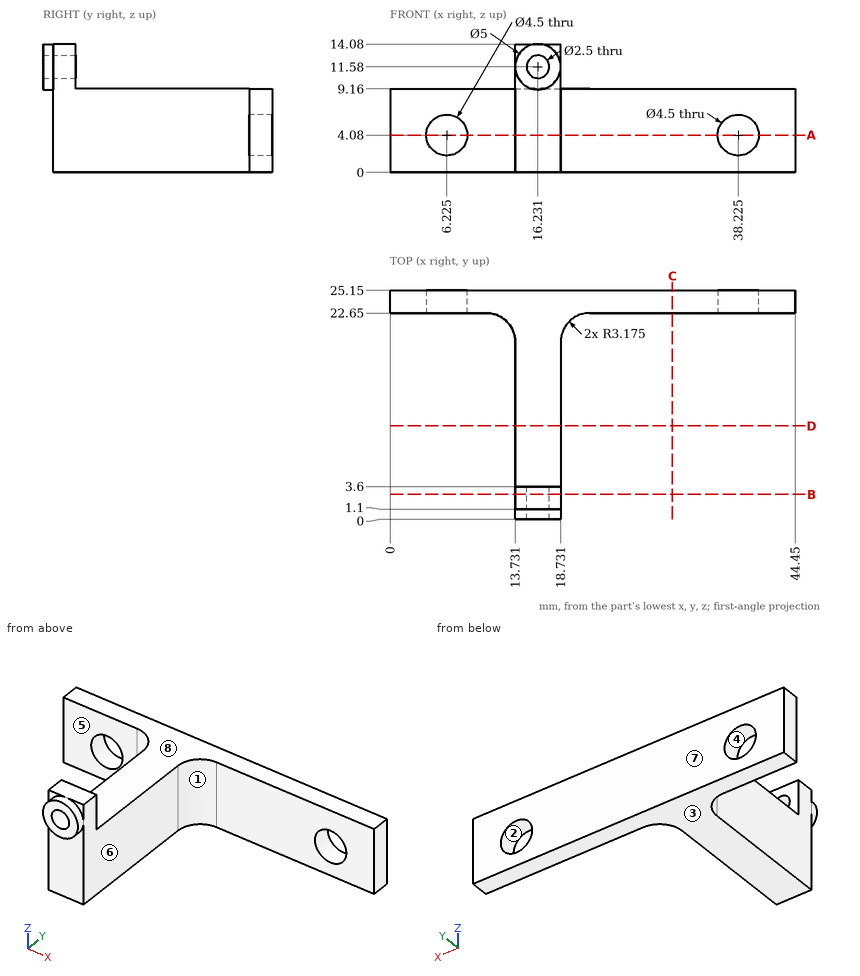
Study the drawing (mm; zero at the part's minimum x, y, z) and answer. A direction names the side the tool comes from. Round coordinates to 2 decimals unless told otherwise and drop trailing zeros. Loops run counter-clockwise (first coordinate to the right, second up) from the corner with the lowest first, then second, coordinate; pieces in that order, holes last.
Q1. Section D-D, the plane y = 10.25 is taken. Determine the outline of the cut face in (x, z).
Q2. Which of the six approach directions +Z, -Z, +X, -X, +Y, -Y give full straight-line access (tool end or side, diameter ignored) to the marked faces 4, 5, 6, 7 and 8?
Q3. Section C-C, the plane x = 31 is taken. Determine the outline of the cut face in (y, z).
Q4. Section A-A, the plane z = 4.08 is taken. Count the separate pieces of the cut face and the enclosed holes in it, then the cut area to 3 significant figures.
Q5. Section B-B, the plane y = 2.75 is taken. Determine the outline of the cut face in (x, z), then the cut area to 3 significant figures.
Q6. Find the intervals of material crossed by line 1 (Y direction, x = 41.5, z = 8.25); line 2 (Z direction, x = 38, y = 23); line 3 (X direction, y = 5, z = 1), in increasing order.
Q7. For a pull along Z with two mould halves and no side action, classify the marked faces 1, 2 and 3 as released by +Z, released by -Z, zero draft, split by the parting line, or undercut.
Q8. Given pin 1 Ø1.5 at (x, z) = (16.23, 11.58) entering from -Y; pin 2 Ø6 at (x, z) = (38.225, 4.08) entering from +Y; pin 3 Ø4 at (x, z) = (16.5, 6.5) entering from -Y; pin 4 Ø7 at (y, z) = (10.5, 4.5) entering from +X, each flat-ended and moving along its own axis, determine where each tip first touches the part or whether it passes through.
Completed:
1. outline: (13.73, 0) - (18.73, 0) - (18.73, 9.16) - (13.73, 9.16) - close
2. face 4: +Y, -Y
2. face 5: +Z, -Z, -X, -Y
2. face 6: +Z, -Z, +X, -Y
2. face 7: +Z, -Z, +X, -X, +Y
2. face 8: +Z, +X, -X, +Y
3. outline: (22.65, 0) - (25.15, 0) - (25.15, 9.16) - (22.65, 9.16) - close
4. separate pieces: 3
4. enclosed holes: 0
4. area: 201 mm2
5. outline: (13.73, 0) - (18.73, 0) - (18.73, 14.08) - (13.73, 14.08) - close; hole circle Ø2.5 at (16.23, 11.58)
5. area: 65.5 mm2
6. line 1: y = 22.65 to 25.15
6. line 2: z = 0 to 1.84, 6.32 to 9.16
6. line 3: x = 13.73 to 18.73
7. face 1: zero draft
7. face 2: undercut
7. face 3: released by -Z
8. pin 1: passes through
8. pin 2: stops at y = 25.15
8. pin 3: stops at y = 1.1
8. pin 4: stops at x = 18.73
